Job drawing, mm, ordinate dimensions from the low corner. One solid piece. A direction names the side the tool comes from. Give positions to 0.01 mm unless a question says otherwise; leave off trailing zeros. Write each loop counter-clockwise with the first axis right and the second up, starting at its lowest first coordinate (ties: lowest second). Pieces come first, ordered by that corner, then holes. Notation, with made-up numbers: (-14.75, 45.25) -> (25.25, 45.25) arc R21 cw to (25.25, 78.25) -> close; hole circle Ø3 at (-38.75, 53). An arc over 180 degrees is marked (long way). One line per question, with ' | ' between items. Start each with the question number.
(1) Band-saw the part on A-A, the plane x = 27. Give the cut face in (y, z), and give its area (3 significant figures).
(2) Band-saw the part on D-D, the plane z = 8. Give the cut face in (x, y).
(3) Tool access for the marked faces 1 and 2: list every direction of +Z, -Z, +X, -X, +Y, -Y with a clear straight run to the whole face (end or side of a thin tool).
(4) Band-saw the part on B-B, the plane x = 49. Count the separate pieces of the cut face and the enclosed holes in it.
(5) Drill centre lines: probe 1 along X at (y, z) = (2.5, 12); probe 2 along X at (y, z) = (12, 51); probe 3 along X at (y, z) = (12.5, 52). Where is each one in solid material? Low to high. Write a range as from..to.
(6) Pin check, flat tips, straight feed: P1, Ø5.5, axis at x = 14, y = 11, coming from the -Z side; P2, Ø8, axis at x = 34, z = 12, coming from the +Y side; P3, Ø5.5, axis at y = 6, z = 16, coming from the -X side. Stop position of each tip, or through.
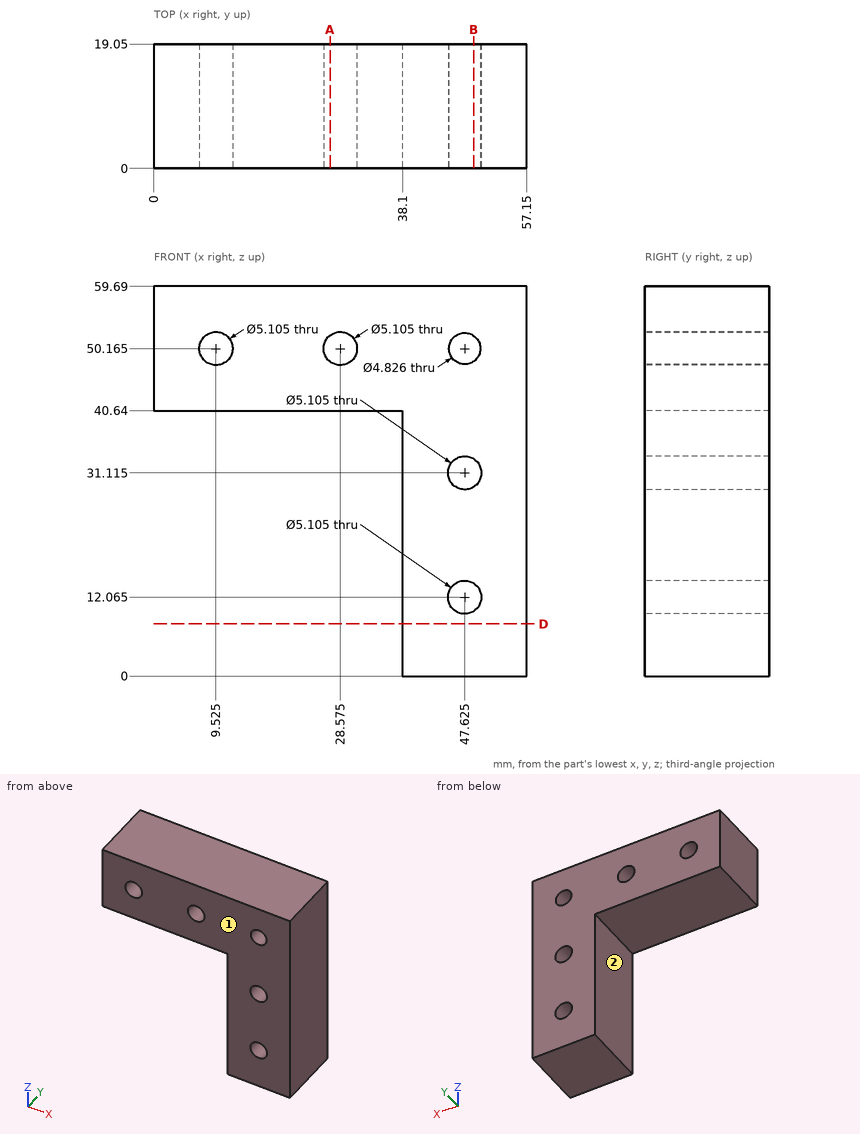
Results:
1) outline: (0, 40.64) -> (19.05, 40.64) -> (19.05, 48.16) -> (0, 48.16) -> close; (0, 52.17) -> (19.05, 52.17) -> (19.05, 59.69) -> (0, 59.69) -> close | area: 286 mm²
2) outline: (38.1, 0) -> (57.15, 0) -> (57.15, 19.05) -> (38.1, 19.05) -> close
3) face 1: +Z, -Z, +X, -X, -Y | face 2: -Z, -X, +Y, -Y
4) separate pieces: 4 | enclosed holes: 0
5) probe 1: x = 38.1..45.07, 50.18..57.15 | probe 2: x = 0..7.11, 11.94..26.16, 30.99..45.36, 49.89..57.15 | probe 3: x = 0..7.75, 11.3..26.8, 30.35..46.06, 49.19..57.15
6) P1: stops at z = 40.64 | P2: passes through | P3: stops at x = 38.1
